```python
from build123d import *

# Parameters (mm, degrees)
CROQUIS2_W              = 43
CROQUIS2_H              = 43
CROQUIS2_R              = 1.6
SALIENTE_EXTRUIR2_DEPTH = 2.5
SALIENTE_EXTRUIR3_DEPTH = 1.5
SALIENTE_EXTRUIR4_DEPTH = 1.5
SALIENTE_EXTRUIR5_DEPTH = 1.5
CROQUIS7_W              = 46
CROQUIS7_H              = 8.5
SALIENTE_EXTRUIR6_DEPTH = 44.5
CROQUIS8_R              = 7.625
CORTAR_EXTRUIR1_DEPTH   = 90.145947749
CROQUIS9_R              = 3
CORTAR_EXTRUIR3_DEPTH   = 16.5
SALIENTE_EXTRUIR8_DEPTH = 1.5
SALIENTE_EXTRUIR9_DEPTH = 1.5
CROQUIS12_R             = 12.25
CUT_EXTRUDE1_DEPTH      = 10
BOSS_EXTRUDE1_DEPTH     = 35
BOSS_EXTRUDE2_START     = -50
SKETCH3_R               = 4.1
BOSS_EXTRUDE2_DEPTH     = 50
BOSS_EXTRUDE3_START     = -3
SKETCH4_R               = 4.1
BOSS_EXTRUDE3_DEPTH     = 3
FILLET1_R               = 4


with BuildPart() as part:
    # Croquis2 → Saliente-Extruir2 (new body)
    with BuildSketch(Plane.XY.offset(-84)):
        Rectangle(CROQUIS2_W, CROQUIS2_H)
        with Locations((-15.511143721, 15.511143721)):
            Circle(CROQUIS2_R, mode=Mode.SUBTRACT)
        with Locations((15.511143721, 15.511143721)):
            Circle(CROQUIS2_R, mode=Mode.SUBTRACT)
        with Locations((15.511143721, -15.511143721)):
            Circle(CROQUIS2_R, mode=Mode.SUBTRACT)
        with Locations((-15.511143721, -15.511143721)):
            Circle(CROQUIS2_R, mode=Mode.SUBTRACT)
    extrude(amount=SALIENTE_EXTRUIR2_DEPTH)

    # Croquis4 → Saliente-Extruir3 (add)
    with BuildSketch(Plane(origin=(0, 21.5, 0), x_dir=(1, 0, 0), z_dir=(0, 1, 0))):
        Polygon((-21.5, 84), (-21.5, 122), (21.5, 122), (21.5, 84), (21.5, 39), (-21.5, 39), align=None)
    extrude(amount=SALIENTE_EXTRUIR3_DEPTH)

    # Croquis5 → Saliente-Extruir4 (add)
    with BuildSketch(Plane.ZY.offset(21.5)):
        Polygon((-60.25, 21.5), (-39, 21.5), (-39, 23), (-122, 23), (-122, 21.5), (-122, -21.5), (-84, -21.5), (-81.5, -21.5), (-81.5, 0), (-81.5, 21.5), align=None)
    extrude(amount=SALIENTE_EXTRUIR4_DEPTH)

    # Croquis6 → Saliente-Extruir5 (add)
    with BuildSketch(Plane(origin=(21.5, 0, 0), x_dir=(0, 0, -1), z_dir=(1, 0, 0))):
        Polygon((122, 21.5), (122, -21.5), (84, -21.5), (81.5, -21.5), (81.5, 0), (81.5, 21.5), (64, 21.5), (39, 21.5), (39, 23), (122, 23), align=None)
    extrude(amount=SALIENTE_EXTRUIR5_DEPTH)

    # Croquis7 → Saliente-Extruir6 (add)
    with BuildSketch(Plane(origin=(0, 23, 0), x_dir=(1, 0, 0), z_dir=(0, 1, 0))):
        with Locations((0, 34.75)):
            Rectangle(CROQUIS7_W, CROQUIS7_H)
    extrude(amount=-SALIENTE_EXTRUIR6_DEPTH)

    # Croquis8 → Cortar-Extruir1 (cut, through all)
    with BuildSketch(Plane(origin=(0, 0, -39), x_dir=(-1, 0, 0), z_dir=(0, 0, -1))):
        Circle(CROQUIS8_R)
    extrude(amount=-CORTAR_EXTRUIR1_DEPTH, mode=Mode.SUBTRACT)

    # Croquis9 → Cortar-Extruir3 (cut)
    with BuildSketch(Plane.XY.offset(-30.5)):
        with Locations((-15.5, 15.5)):
            Circle(CROQUIS9_R)
        with Locations((15.5, 15.5)):
            Circle(CROQUIS9_R)
        with Locations((-15.5, -15.5)):
            Circle(CROQUIS9_R)
        with Locations((15.5, -15.5)):
            Circle(CROQUIS9_R)
    extrude(amount=-CORTAR_EXTRUIR3_DEPTH, mode=Mode.SUBTRACT)

    # Croquis10 → Saliente-Extruir8 (add)
    with BuildSketch(Plane.ZY.offset(23)):
        Polygon((-39, -21.5), (-39, 21.5), (-81.5, 21.5), (-81.5, 0), (-81.5, -21.5), align=None)
    extrude(amount=-SALIENTE_EXTRUIR8_DEPTH)

    # Croquis11 → Saliente-Extruir9 (add)
    with BuildSketch(Plane(origin=(23, 0, 0), x_dir=(0, 0, -1), z_dir=(1, 0, 0))):
        Polygon((39, 21.5), (81.5, 21.5), (81.5, 0), (81.5, -21.5), (39, -21.5), align=None)
    extrude(amount=-SALIENTE_EXTRUIR9_DEPTH)

    # Croquis12 → Cut-Extrude1 (cut)
    with BuildSketch(Plane.XY.offset(-81.5)):
        Circle(CROQUIS12_R)
    extrude(amount=-CUT_EXTRUDE1_DEPTH, mode=Mode.SUBTRACT)

    # Sketch2 → Boss-Extrude1 (add)
    with BuildSketch(Plane.XY.offset(-30.5)):
        with BuildLine():
            Line((-37.67617907, 1), (-37.67617907, 3))
            Line((-37.67617907, 3), (-33.01130869, 3))
            ThreePointArc((-33.01130869, 3), (-28.23921976, 6.076120641), (-23, 3.888444419))
            Line((-23, 3.888444419), (-23, -3.888444419))
            ThreePointArc((-23, -3.888444419), (-28.23921976, -6.076120641), (-33.01130869, -3))
            Line((-33.01130869, -3), (-37.67617907, -3))
            Line((-37.67617907, -3), (-37.67617907, -1))
            Line((-37.67617907, -1), (-31.67617907, -1))
            ThreePointArc((-31.67617907, -1), (-23.6, 0), (-31.67617907, 1))
            Line((-31.67617907, 1), (-37.67617907, 1))
        make_face()
        with BuildLine():
            Line((23, 3.888444419), (23, -3.888444419))
            ThreePointArc((23, -3.888444419), (28.23921976, -6.076120641), (33.01130869, -3))
            Line((33.01130869, -3), (37.67617907, -3))
            Line((37.67617907, -3), (37.67617907, -1))
            Line((37.67617907, -1), (31.67617907, -1))
            ThreePointArc((31.67617907, -1), (23.6, 0), (31.67617907, 1))
            Line((31.67617907, 1), (37.67617907, 1))
            Line((37.67617907, 1), (37.67617907, 3))
            Line((37.67617907, 3), (33.01130869, 3))
            ThreePointArc((33.01130869, 3), (28.23921976, 6.076120641), (23, 3.888444419))
        make_face()
    extrude(amount=-BOSS_EXTRUDE1_DEPTH)

    # Sketch3 → Boss-Extrude2 (add)
    # profile 1 of 2: a face of its own
    with BuildSketch(Plane(origin=(0, 0, -122), x_dir=(-1, 0, 0), z_dir=(0, 0, -1)).offset(BOSS_EXTRUDE2_START)):
        with BuildLine():
            Line((-23, -4.489988864), (-23, 4.489988864))
            ThreePointArc((-23, 4.489988864), (-34.2, 0), (-23, -4.489988864))
        make_face()
        with Locations((-27.7, 0)):
            Circle(SKETCH3_R, mode=Mode.SUBTRACT)
    # profile 2 of 2: a face of its own
    with BuildSketch(Plane(origin=(0, 0, -122), x_dir=(-1, 0, 0), z_dir=(0, 0, -1)).offset(BOSS_EXTRUDE2_START)):
        with BuildLine():
            ThreePointArc((23, -4.489988864), (34.2, 0), (23, 4.489988864))
            Line((23, 4.489988864), (23, -4.489988864))
        make_face()
        with Locations((27.7, 0)):
            Circle(SKETCH3_R, mode=Mode.SUBTRACT)
    extrude(amount=BOSS_EXTRUDE2_DEPTH)

    # Sketch4 → Boss-Extrude3 (add)
    with BuildSketch(Plane(origin=(0, 0, -122), x_dir=(-1, 0, 0), z_dir=(0, 0, -1)).offset(BOSS_EXTRUDE3_START)):
        with Locations((-27.7, 0)):
            Circle(SKETCH4_R)
        with Locations((27.7, 0)):
            Circle(SKETCH4_R)
    extrude(amount=BOSS_EXTRUDE3_DEPTH)

    # Fillet1
    fillet1_edges = [part.edges().sort_by_distance(p)[0] for p in [
        (-23, 3.888444419, -48),
        (-23, -3.888444419, -48),
        (23, 3.888444419, -48),
        (23, -3.888444419, -48),
        (23, 4.489988864, -97),
        (23, -4.489988864, -97),
        (-23, -4.489988864, -97),
        (-23, 4.489988864, -97),
    ]]
    fillet(fillet1_edges, radius=FILLET1_R)


solid = part.part
```
Work out the finished part from the listing and answer in its coordinate system (mm). A direction names the side the tool comes from. Give positions to 0.01 mm unless a question says otherwise; leave off trailing zeros. Loops run counter-clockwise (first coordinate to the right, second up) from the corner with the lowest first, then second, coordinate; pieces in that order, holes last. Notation, with made-up numbers: (44, 80) -> (53, 80) arc R9 ccw to (53, 87) -> close; hole circle Ø1 at (89.5, 67.25). An arc over 180 degrees is marked (long way). Use CSV: the item, a comma, the result in double quotes.
1. The part is cut by section C-C (x = 15.5). Write down the section's boundary in (y, z).
Found:
outline,"(-21.5, -84) -> (-17.11, -84) -> (-17.11, -81.5) -> (-21.5, -81.5) -> close; (-21.5, -39) -> (-18.5, -39) -> (-18.5, -30.5) -> (-21.5, -30.5) -> close; (-13.91, -84) -> (13.91, -84) -> (13.91, -81.5) -> (-13.91, -81.5) -> close; (-12.5, -39) -> (12.5, -39) -> (12.5, -30.5) -> (-12.5, -30.5) -> close; (17.11, -84) -> (21.5, -84) -> (21.5, -122) -> (23, -122) -> (23, -30.5) -> (18.5, -30.5) -> (18.5, -39) -> (21.5, -39) -> (21.5, -81.5) -> (17.11, -81.5) -> close"
2. Flat-ended cylindrical pins translate along their axes: pin 1 Ø6.5 at (x, z) = (34.5, -55.5) entering from +Y; pin 2 Ø4 at (x, y) = (28, 1) entering from +Z; pin 3 Ø4 at (y, z) = (-11, -52) entering from +X; pin 4 Ø10 at (x, y) = (-4, 2.5) entering from +Z. Find the tip coordinate at first contact, or state that the pin passes through.
Found:
pin 1,"y = 4.96"
pin 2,"z = -119"
pin 3,"x = 23.15"
pin 4,"z = -30.5"
3. The mould has two halves that part along Z. Classify faces 1 (the flat face through (37.676, -2, -48)), 2 (the flat face through (8, 1, -30.5)), 3 (the flat face through (-31.4, -2.2, -65.5)): +Z half, -Z half, draft (parallel to the pull), parting line (faces both ways), or undercut.
Found:
face 1,"draft"
face 2,"+Z half"
face 3,"undercut"
4. A tool of negligible diameter and unlimited length cuts with its end or side. For faces 4 (the flat face through (0, 21.5, -103)), 5 (the cylindrical face through (6.586, 10.329, -82.732)), 6 (the flat face through (35, -1, -48)), 7 (the flat face through (-21.5, 0, -61)), 8 (the cylindrical face through (23.603, -0.166, -47.755)), from which of +Z, -Z, +X, -X, +Y, -Y can it reach the whole face along a straight path? Write none if from no direction.
Found:
face 4,"-Z, -Y"
face 5,"-Z"
face 6,"+Z, +X"
face 7,"-Y"
face 8,"+Z"
5. The part is cut by section B-B (z = -77). Write down the section's boundary in (x, y).
Found:
outline,"(-27.27, -6.49) arc R4 cw to (-23, -10.48) -> (-23, -21.5) -> (-21.5, -21.5) -> (-21.5, 21.5) -> (21.5, 21.5) -> (21.5, -21.5) -> (23, -21.5) -> (23, -10.48) arc R4 cw to (27.27, -6.49) arc R6.5 ccw (long way) to (27.27, 6.49) arc R4 cw to (23, 10.48) -> (23, 23) -> (-23, 23) -> (-23, 10.48) arc R4 cw to (-27.27, 6.49) arc R6.5 ccw (long way) to start; hole circle Ø8.2 at (-27.7, 0); hole circle Ø8.2 at (27.7, 0)"
6. Straight lines are drawn through the part: line 1 (Y direction, x = -15.5, z = -35.25); line 2 (X direction, y = 4.5, z = -60); line 3 (Z direction, x = -12.5, y = 12). For each, find the intervals that lie inside material, in ascending order.
Found:
line 1,"-21.5 to -18.5, -12.5 to 12.5, 18.5 to 23"
line 2,"-31.82 to -21.5, 21.5 to 31.82"
line 3,"-84 to -81.5, -39 to -30.5"
7. The part is cut by section A-A (x = 0). Write down the section's boundary in (y, z) (3 decimals).
Found:
outline,"(-21.5, -84) -> (-12.25, -84) -> (-12.25, -81.5) -> (-21.5, -81.5) -> close; (-21.5, -39) -> (-7.625, -39) -> (-7.625, -30.5) -> (-21.5, -30.5) -> close; (7.625, -39) -> (21.5, -39) -> (21.5, -81.5) -> (12.25, -81.5) -> (12.25, -84) -> (21.5, -84) -> (21.5, -122) -> (23, -122) -> (23, -30.5) -> (7.625, -30.5) -> close"
